```python
from build123d import *

# Parameters (mm, degrees)
ESQUISSE1_W             = 25.4
ESQUISSE1_H             = 12.7
BOSS_EXTRU_1_DEPTH      = 6.35
BOSS_EXTRU_2_DEPTH      = 12.7
CONG_1_R                = 1.27
ESQUISSE3_R             = 1.5
ENL_V_MAT_EXTRU_1_DEPTH = 9.525


with BuildPart() as part:
    # Esquisse1 → Boss.-Extru.1 (new body)
    with BuildSketch(Plane.XY):
        Rectangle(ESQUISSE1_W, ESQUISSE1_H)
    extrude(amount=BOSS_EXTRU_1_DEPTH)

    # Esquisse2 → Boss.-Extru.2 (add)
    with BuildSketch(Plane.XZ.offset(6.35)):
        with BuildLine():
            Line((-12.7, 6.35), (-27.474417663, 23.102614958))
            ThreePointArc((-27.474417663, 23.102614958), (-27.500391754, 24.752263413), (-25.875041622, 25.035550597))
            ThreePointArc((-25.875041622, 25.035550597), (0, 17.951934494), (25.875041622, 25.035550597))
            ThreePointArc((25.875041622, 25.035550597), (27.500391754, 24.752263413), (27.474417663, 23.102614958))
            Line((27.474417663, 23.102614958), (12.7, 6.35))
            Line((12.7, 6.35), (12.7, 0))
            Line((12.7, 0), (-12.7, 0))
            Line((-12.7, 0), (-12.7, 6.35))
        make_face()
    extrude(amount=-BOSS_EXTRU_2_DEPTH)

    # Congé1
    cong_1_edges = [part.edges().sort_by_distance(p)[0] for p in [
        (-12.7, 0, 6.35),
        (-20.087208832, 6.35, 14.726307479),
        (-27.500391754, 6.35, 24.752263413),
        (0, 6.35, 17.951934494),
        (27.500391754, 6.35, 24.752263413),
        (20.087208832, 6.35, 14.726307479),
        (20.087208832, -6.35, 14.726307479),
        (27.500391754, -6.35, 24.752263413),
        (0, -6.35, 17.951934494),
        (-27.500391754, -6.35, 24.752263413),
        (-20.087208832, -6.35, 14.726307479),
        (12.7, 0, 6.35),
        (12.7, -6.35, 3.175),
        (-12.7, -6.35, 3.175),
        (-12.7, 6.35, 3.175),
        (12.7, 6.35, 3.175),
    ]]
    fillet(cong_1_edges, radius=CONG_1_R)

    # Esquisse3 → Enlèv. mat.-Extru.1 (cut)
    with BuildSketch(Plane(origin=(0, 0, 0), x_dir=(-1, 0, 0), z_dir=(0, 0, -1))):
        with Locations((-6.35, 0)):
            Circle(ESQUISSE3_R)
        with Locations((6.35, 0)):
            Circle(ESQUISSE3_R)
    extrude(amount=-ENL_V_MAT_EXTRU_1_DEPTH, mode=Mode.SUBTRACT)


solid = part.part
```
CAD build for the part. Positions are in the model's coordinates, mm. A direction names the side the tool comes from. Round coordinates to 2 decimals unless told otherwise and drop trailing zeros. Write each loop counter-clockwise with the first axis right and the second up, starting at its lowest first coordinate (ties: lowest second). Pieces come first, ordered by that corner, then holes. Notation, with made-up numbers: (-15, 40.25) - (9, 40.25) arc R15 cw to (9, 47.25) - close; hole circle Ø7 at (89, 32). An arc over 180 degrees is marked (long way). Write item = value, one per line. Start each with the question number.
Q1. Band-saw the part on B-B (y = 4.5). Give the cut face in (x, z).
Q2. Probe L1, parallel to Y at x = 6.35, z = 2.25; L2, parallel to X at y = 3.75, z = 1.5; L3, parallel to X at y = 0.75, z = 7.25. List the from-to ranges inside material, lowest first. Write a range as from..to.
Q3. Band-saw the part on C-C (y = 0.75). Give the cut face in (x, z) (1 decimal), then the cut area to 3 significant figures.
Q4. Drop flat-ended pins along their axis: pin 1 (2.5 mm diameter, centred on x = -6.35, y = 0, fed in from +Z); pin 2 (4.5 mm diameter, centred on y = 0.5, z = 4.5, fed in from -X); pin 3 (0.9 mm diameter, centred on x = 6.5, y = -0.5, fed in from -Z) (3 decimals). Give the stop position or say it passes through.
Q5. Band-saw the part on A-A (z = 2.5). Give the cut face in (x, y).
Q6. Mould opens along Y. For faces 1 (the flat face through (6, 0, 9.525)), 2 (the cylindrical face through (-12.338, -5.968, 2.976)), 3 (the flat face through (20.347, -0.071, 15.021)), 4 (the cylindrical face through (19.87, 5.97, 15.03)) say: pulls with the +Y half, pulls with the -Y half, needs draft (parallel to the pull), parting line crosses it, or undercut.
Q7. Which spindle directions (+Z, -Z, +X, -X, +Y, -Y) get a long thin tool onto all of the face, cutting with end or side? Do faces 5 (the flat face through (-12.7, 0, 3)), 6 (the flat face through (12.7, 0, 3)), 7 (the cylindrical face through (12.318, -5.988, 2.976)). Say none if no direction does.
Answers below:
q1.outline = (-27.47, 23.1) - (-13.02, 6.71) arc R1.27 cw to (-12.7, 5.87) - (-12.7, 0) - (12.7, 0) - (12.7, 5.87) arc R1.27 cw to (13.02, 6.71) - (27.47, 23.1) arc R1.27 ccw to (25.88, 25.04) arc R50.8 cw to (-25.88, 25.04) arc R1.27 ccw to start
q2.L1 = -6.35..-1.5, 1.5..6.35
q2.L2 = -12.7..12.7
q2.L3 = -13.49..-7.65, -5.05..5.05, 7.65..13.49
q3.outline = (-27.5, 23.1) - (-13, 6.7) arc R1.3 cw to (-12.7, 5.9) - (-12.7, 0) - (-7.6, 0) - (-7.6, 9.5) - (-5.1, 9.5) - (-5.1, 0) - (5.1, 0) - (5.1, 9.5) - (7.6, 9.5) - (7.6, 0) - (12.7, 0) - (12.7, 5.9) arc R1.3 cw to (13, 6.7) - (27.5, 23.1) arc R1.3 ccw to (25.9, 25) arc R50.8 cw to (-25.9, 25) arc R1.3 ccw to start
q3.area = 644 mm2
q4.pin_1 = 18.52
q4.pin_2 = -13.05
q4.pin_3 = 9.525
q5.outline = (-12.7, -5.08) arc R1.27 ccw to (-11.43, -6.35) - (11.43, -6.35) arc R1.27 ccw to (12.7, -5.08) - (12.7, 5.08) arc R1.27 ccw to (11.43, 6.35) - (-11.43, 6.35) arc R1.27 ccw to (-12.7, 5.08) - close; hole circle Ø3 at (-6.35, 0); hole circle Ø3 at (6.35, 0)
q6.face_1 = undercut
q6.face_2 = pulls with the -Y half
q6.face_3 = needs draft
q6.face_4 = pulls with the +Y half
q7.face_5 = -Z, -X, +Y, -Y
q7.face_6 = -Z, +X, +Y, -Y
q7.face_7 = -Z, +X, -Y
